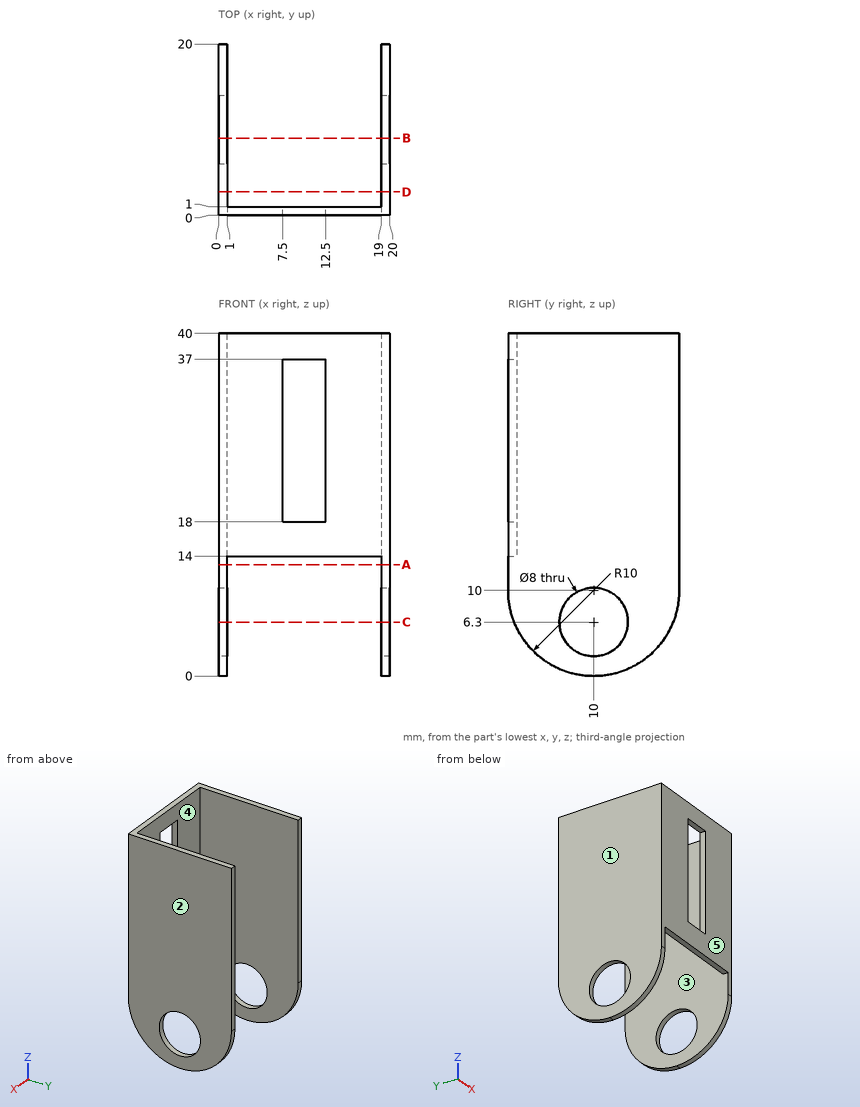
The figure shows three views and two pictorial views of one solid part (mm, origin at its lowest corner). Answer the questions. A direction names the side the tool comes from. Round coordinates to 2 decimals unless told otherwise and drop trailing zeros. Loops run counter-clockwise (first coordinate to the right, second up) from the corner with the lowest first, then second, coordinate; pieces in that order, holes last. Notation, with made-up numbers: (-16.75, 41.25) - (8.25, 41.25) arc R14 ccw to (8.25, 66.25) - close; hole circle Ø10 at (32, 56.5). An arc over 180 degrees is marked (long way). One line per question, with ' | ' between items. Start each with the question number.
Q1. For a pull along X with two mould halves and no side action, classify the marked faces 1, 2 and 3 as +X half, -X half, draft (parallel to the pull), parting line (faces both ways), or undercut.
Q2. Flat-ended cylindrical pins translate along their axes: pin 1 (0.8 mm diameter, centred on y = 0.5, z = 30, fed in from -X); pin 2 (0.8 mm diameter, centred on x = 10.5, y = 0.5, fed in from -Z); pin 3 (8 mm diameter, centred on x = 9, z = 8.5, fed in from -Y). Find the tip coordinate at first contact, or state that the pin passes through.
Q3. Find the intervals of material crossed by L1, parallel to X at y = 3.5, z = 29.5; L2, parallel to Y at x = 2.75, z = 28; L3, parallel to Y at x = 0.75, z = 6.3, in increasing order.
Q4. Section C-C on z = 6.3 is taken. Give the vertices of the cut face in (x, y), plus the area to 3 significant figures.
Q5. Section D-D on y = 2.75 is taken. Give the vertices of the cut face in (x, z), plus the area to 3 significant figures.
Q6. Section A-A on z = 13 is taken. Give the vertices of the cut face in (x, y), plus the area to 3 significant figures.
Q7. Section B-B on y = 9 is taken. Give the vertices of the cut face in (x, z), plus the area to 3 significant figures.
Q8. For the marked faces 4 and 5, determine the directions among +Z, -Z, +X, -X, +Y, -Y from which every point of the face is accessible in a straight line to the end or side of a thin tool.
Established:
1) face 1: -X half | face 2: +X half | face 3: undercut
2) pin 1: x = 0 | pin 2: z = 14 | pin 3: through
3) L1: 0 to 1, 19 to 20 | L2: 0 to 1 | L3: 0.71 to 6, 14 to 19.29
4) outline: (0, 0.71) - (1, 0.71) - (1, 6) - (0, 6) - close; (0, 14) - (1, 14) - (1, 19.29) - (0, 19.29) - close; (19, 0.71) - (20, 0.71) - (20, 6) - (19, 6) - close; (19, 14) - (20, 14) - (20, 19.29) - (19, 19.29) - close | area: 21.2 mm²
5) outline: (0, 3.11) - (1, 3.11) - (1, 40) - (0, 40) - close; (19, 3.11) - (20, 3.11) - (20, 40) - (19, 40) - close | area: 73.8 mm²
6) outline: (0, 0) - (1, 0) - (1, 20) - (0, 20) - close; (19, 0) - (20, 0) - (20, 20) - (19, 20) - close | area: 40.0 mm²
7) outline: (0, 0.05) - (1, 0.05) - (1, 2.43) - (0, 2.43) - close; (0, 10.17) - (1, 10.17) - (1, 40) - (0, 40) - close; (19, 0.05) - (20, 0.05) - (20, 2.43) - (19, 2.43) - close; (19, 10.17) - (20, 10.17) - (20, 40) - (19, 40) - close | area: 64.4 mm²
8) face 4: +Z, -Z, +Y | face 5: +Z, -Z, +X, -X, -Y
